The model under review builds one solid part; all positions refer to its coordinate system, in mm. Round coordinates to 2 decimals unless told otherwise and drop trailing zeros. Loops run counter-clockwise (first coordinate to the right, second up) from the corner with the lowest first, then second, coordinate; pieces in that order, holes last. Notation, with made-up numbers: M 6,55.5 L 60,55.5 A23 ccw 60,91.5 Z; hole C -13.5,68.25 d8. An arc over 180 degrees is marked long. One line per question, with ' | ' between items.
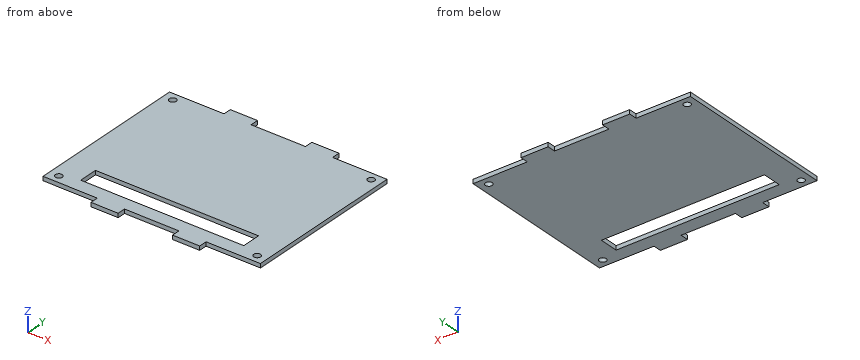
from build123d import *

# Parameters (mm, degrees)
F0_R     = 2.5
F1_DEPTH = 1.5


with BuildPart() as f1:
    # F0 (on Top) → F1 (new body, symmetric)
    with BuildSketch(Plane.XY):
        Polygon((80, -60), (80, 60), (40, 60), (40, 66), (20, 66), (20, 60), (-20, 60), (-20, 66), (-40, 66), (-40, 60), (-80, 60), (-80, -60), (-40, -60), (-40, -66), (-20, -66), (-20, -60), (20, -60), (20, -66), (40, -66), (40, -60), align=None)
        with Locations((-73, -54)):
            Circle(F0_R, mode=Mode.SUBTRACT)
        Polygon((60, -50), (0, -50), (-60, -50), (-60, -36), (60, -36), align=None, mode=Mode.SUBTRACT)
        with Locations((73, -54)):
            Circle(F0_R, mode=Mode.SUBTRACT)
        with Locations((-73, 54)):
            Circle(F0_R, mode=Mode.SUBTRACT)
        with Locations((73, 54)):
            Circle(F0_R, mode=Mode.SUBTRACT)
    extrude(amount=F1_DEPTH, both=True)


solid = f1.part
1) Add section B-B on y = 54. State the section outline as (x, z) points, then the cut area to 3 significant figures.
Output values:
outline: M -80,-1.5 L -75.5,-1.5 L -75.5,1.5 L -80,1.5 Z; M -70.5,-1.5 L 70.5,-1.5 L 70.5,1.5 L -70.5,1.5 Z; M 75.5,-1.5 L 80,-1.5 L 80,1.5 L 75.5,1.5 Z | area: 450 mm²
2) Add section A-A on x = 23. State the section outline as (y, z) points.
Output values:
outline: M -66,-1.5 L -50,-1.5 L -50,1.5 L -66,1.5 Z; M -36,-1.5 L 66,-1.5 L 66,1.5 L -36,1.5 Z
3) For line 1 (Y direction, x = -73, z = 0.8); line 2 (Y direction, x = -39.5, z = -0.75); line 3 (Y direction, x = -7.5, z = -0.1), list the stretches that pass through material, from the lowest coordinate up.
Output values:
line 1: y = -60 to -56.5, -51.5 to 51.5, 56.5 to 60 | line 2: y = -66 to -50, -36 to 66 | line 3: y = -60 to -50, -36 to 60
4) Add section C-C on x = 73. State the section outline as (y, z) points, then the cut area to 3 significant figures.
Output values:
outline: M -60,-1.5 L -56.5,-1.5 L -56.5,1.5 L -60,1.5 Z; M -51.5,-1.5 L 51.5,-1.5 L 51.5,1.5 L -51.5,1.5 Z; M 56.5,-1.5 L 60,-1.5 L 60,1.5 L 56.5,1.5 Z | area: 330 mm²
5) Add section D-D on z = -0.55. State the section outline as (x, y) points.
Output values:
outline: M -80,-60 L -40,-60 L -40,-66 L -20,-66 L -20,-60 L 20,-60 L 20,-66 L 40,-66 L 40,-60 L 80,-60 L 80,60 L 40,60 L 40,66 L 20,66 L 20,60 L -20,60 L -20,66 L -40,66 L -40,60 L -80,60 Z; hole C -73,-54 d5; hole C -73,54 d5; hole M -60,-50 L 60,-50 L 60,-36 L -60,-36 Z; hole C 73,-54 d5; hole C 73,54 d5
6) Insertion check: P1, Ø0.9, axis at y = 64, z = -0.5, coming from the -X side; P2, Ø0.9, axis at y = -64, z = 0, coming from the +X side; P3, Ø0.9, axis at x = -66, z = 0, coming from the -Y side; P4, Ø8, axis at x = -73, y = -54, coming from the -Z side. Each pin has a flat end and moves straight along its axis. Give the tip position at first contact, or say it passes through.
Output values:
P1: stops at x = -40 | P2: stops at x = 40 | P3: stops at y = -60 | P4: stops at z = -1.5
